from build123d import *

# Parameters (mm, degrees)
BOSS_EXTRUDE1_DEPTH     = 40
CUT_EXTRUDE1_DEPTH      = 13
CUT_EXTRUDE1_DEPTH_BACK = 50
SKETCH12_R              = 1.150000001
SKETCH14_R              = 1.150000001
CUT_EXTRUDE2_DEPTH      = 50
SKETCH15_R              = 1.150000001
CUT_EXTRUDE3_DEPTH      = 50
SKETCH18_R              = 7.063467882
CUT_EXTRUDE6_DEPTH      = 50
CUT_EXTRUDE8_DEPTH      = 50
CUT_EXTRUDE8_DEPTH_BACK = 50
SKETCH19_R              = 1.6
SKETCH19_R_2            = 2.999999999


with BuildPart() as part:
    # Sketch9 → Boss-Extrude1 (new body)
    with BuildSketch(Plane(origin=(23635.895639599, 0, 0), x_dir=(0, 0, -1), z_dir=(1, 0, 0))):
        with BuildLine():
            Line((44.099999999, 2015.086397777), (44.099999999, 2022.286397779))
            Line((44.099999999, 2022.286397779), (42.3, 2022.286397779))
            Line((42.3, 2022.286397779), (42.3, 2015.286397778))
            ThreePointArc((42.3, 2015.286397778), (42.007106781, 2014.579290998), (41.300000001, 2014.286397779))
            Line((41.300000001, 2014.286397779), (2.800000001, 2014.286397779))
            ThreePointArc((2.800000001, 2014.286397779), (2.092893219, 2014.579290997), (1.799999999, 2015.286397778))
            Line((1.799999999, 2015.286397778), (1.799999999, 2022.286397779))
            Line((1.799999999, 2022.286397779), (0, 2022.286397779))
            Line((0, 2022.286397779), (0, 2015.086397777))
            ThreePointArc((0, 2015.086397777), (0.761522369, 2013.247920146), (2.599999999, 2012.486397778))
            Line((2.599999999, 2012.486397778), (41.5, 2012.486397778))
            ThreePointArc((41.5, 2012.486397778), (43.33847763, 2013.247920146), (44.099999999, 2015.086397777))
        make_face()
    extrude(amount=-BOSS_EXTRUDE1_DEPTH)

    # Sketch12 → Cut-Extrude1 (cut, two sides: drawn at the far end of the back side and taken through both)
    with BuildSketch(Plane.XY.offset(-CUT_EXTRUDE1_DEPTH_BACK)):
        with Locations(Location((23613.365202112, 2019.805962196, 0), (0, 0, 180))):
            Circle(SKETCH12_R)
    extrude(amount=CUT_EXTRUDE1_DEPTH + CUT_EXTRUDE1_DEPTH_BACK, mode=Mode.SUBTRACT)

    # Sketch14 → Cut-Extrude2 (cut)
    with BuildSketch(Plane.XY):
        with Locations((23605.845202113, 2020.305962197)):
            Circle(SKETCH14_R)
    extrude(amount=-CUT_EXTRUDE2_DEPTH, mode=Mode.SUBTRACT)

    # Sketch15 → Cut-Extrude3 (cut)
    with BuildSketch(Plane.XY):
        with Locations((23598.365202112, 2019.805962196)):
            Circle(SKETCH15_R)
    extrude(amount=-CUT_EXTRUDE3_DEPTH, mode=Mode.SUBTRACT)

    # Sketch18 → Cut-Extrude6 (cut)
    with BuildSketch(Plane.XY):
        with Locations((23625.865202113, 2027.305962196)):
            Circle(SKETCH18_R)
    extrude(amount=-CUT_EXTRUDE6_DEPTH, mode=Mode.SUBTRACT)

    # Sketch19 → Cut-Extrude8 (cut, two sides: drawn at the far end of the back side and taken through both)
    with BuildSketch(Plane(origin=(0, 2012.486397778, 0), x_dir=(-1, 0, 0), z_dir=(0, 1, 0)).offset(-CUT_EXTRUDE8_DEPTH_BACK)):
        with Locations(Location((-23605.996144663, -8.550000002, 0), (0, 0, 269.999999999))):
            Circle(SKETCH19_R)
        with Locations(Location((-23615.895639599, -8.550000002, 0), (0, 0, 269.999999999))):
            Circle(SKETCH19_R)
        with Locations(Location((-23625.795134534, -8.550000002, 0), (0, 0, 269.999999999))):
            Circle(SKETCH19_R)
        with Locations(Location((-23630.744882003, -17.100252533, 0), (0, 0, 270))):
            Circle(SKETCH19_R)
        with Locations(Location((-23620.845387068, -17.100252533, 0), (0, 0, 269.999999999))):
            Circle(SKETCH19_R)
        with Locations(Location((-23610.94589213, -17.100252533, 0), (0, 0, 269.999999999))):
            Circle(SKETCH19_R)
        with Locations(Location((-23601.046397194, -17.100252533, 0), (0, 0, 269.999999999))):
            Circle(SKETCH19_R)
        with Locations(Location((-23601.046397194, -26.999747469, 0), (0, 0, 269.999999999))):
            Circle(SKETCH19_R)
        with Locations(Location((-23610.94589213, -26.999747469, 0), (0, 0, 269.999999999))):
            Circle(SKETCH19_R)
        with Locations(Location((-23620.845387068, -26.999747469, 0), (0, 0, 269.999999999))):
            Circle(SKETCH19_R)
        with Locations(Location((-23630.744882003, -26.999747469, 0), (0, 0, 270))):
            Circle(SKETCH19_R)
        with Locations(Location((-23625.795134534, -35.550000002, 0), (0, 0, 269.999999999))):
            Circle(SKETCH19_R)
        with Locations(Location((-23615.895639599, -35.550000002, 0), (0, 0, 269.999999999))):
            Circle(SKETCH19_R)
        with Locations(Location((-23605.996144663, -35.550000002, 0), (0, 0, 269.999999999))):
            Circle(SKETCH19_R)
        with Locations(Location((-23615.895639599, -22.050000002, 0), (0, 0, 270))):
            Circle(SKETCH19_R_2)
        with Locations(Location((-23625.795134534, -22.050000002, 0), (0, 0, 270))):
            Circle(SKETCH19_R_2)
        with Locations(Location((-23605.996144663, -22.050000002, 0), (0, 0, 269.999999999))):
            Circle(SKETCH19_R_2)
    extrude(amount=CUT_EXTRUDE8_DEPTH + CUT_EXTRUDE8_DEPTH_BACK, mode=Mode.SUBTRACT)


solid = part.part
Model file for the job. Use its own axes, mm. A direction names the side the tool comes from. Give positions to 0.01 mm unless a question says otherwise; leave off trailing zeros. Order: outer loops, then holes, each group sorted by start corner. A loop starts at its lowest first (then second) coordinate and runs counter-clockwise, first axis right, second up. Notation, with made-up numbers: M -8,29 L 10,29 A38 ccw 10,68 Z; hole C 57,-19.5 d3. An arc over 180 degrees is marked long. Write item = value, one per line.
Q1. Cut at B-B, the plane y = 2016.5. List the corners of the cut face in (x, z).
Derived:
outline = M 23595.9,-44.1 L 23635.9,-44.1 L 23635.9,-42.3 L 23595.9,-42.3 Z; M 23595.9,-1.8 L 23635.9,-1.8 L 23635.9,0 L 23595.9,0 Z
Q2. Cut at C-C, the plane x = 23600.5. List the corners of the cut face in (y, z), then the cut area to 3 significant figures.
Derived:
outline = M 2012.49,-41.5 A2.6 ccw 2015.09,-44.1 L 2022.29,-44.1 L 2022.29,-42.3 L 2015.29,-42.3 A1 cw 2014.29,-41.3 L 2014.29,-28.5 L 2012.49,-28.5 Z; M 2012.49,-25.5 L 2014.29,-25.5 L 2014.29,-18.6 L 2012.49,-18.6 Z; M 2012.49,-15.6 L 2014.29,-15.6 L 2014.29,-2.8 A1 cw 2015.29,-1.8 L 2022.29,-1.8 L 2022.29,0 L 2015.09,0 A2.6 ccw 2012.49,-2.6 Z
area = 94.9 mm2
Q3. Cut at A-A, the plane z = -35.55. List the corners of the cut face in (x, y).
Derived:
outline = M 23595.9,2012.49 L 23604.4,2012.49 L 23604.4,2014.29 L 23595.9,2014.29 Z; M 23607.6,2012.49 L 23614.3,2012.49 L 23614.3,2014.29 L 23607.6,2014.29 Z; M 23617.5,2012.49 L 23624.2,2012.49 L 23624.2,2014.29 L 23617.5,2014.29 Z; M 23627.4,2012.49 L 23635.9,2012.49 L 23635.9,2014.29 L 23627.4,2014.29 Z
Q4. Drill centre lines: line 1 (X direction, y = 2013.4, z = -8.55); line 2 (X direction, y = 2013, z = -22.05); line 3 (Z direction, x = 23610, y = 2018.75). Where is each one in solid material? Low to high. Write a range as [from, to].
Derived:
line_1 = [23595.9, 23604.4], [23607.6, 23614.3], [23617.5, 23624.2], [23627.4, 23635.9]
line_2 = [23595.9, 23603], [23609, 23612.9], [23618.9, 23622.8], [23628.8, 23635.9]
line_3 = [-44.1, -42.3], [-1.8, 0]
Q5. Cut at D-D, the plane x = 23618. List the corners of the cut face in (y, z), then the cut area to 3 significant figures.
Derived:
outline = M 2012.49,-41.5 A2.6 ccw 2015.09,-44.1 L 2022.29,-44.1 L 2022.29,-42.3 L 2015.29,-42.3 A1 cw 2014.29,-41.3 L 2014.29,-24.19 L 2012.49,-24.19 Z; M 2012.49,-19.91 L 2014.29,-19.91 L 2014.29,-2.8 A1 cw 2015.29,-1.8 L 2022.29,-1.8 L 2022.29,0 L 2015.09,0 A2.6 ccw 2012.49,-2.6 Z
area = 98.0 mm2
Q6. Tool access for faces 1 (the cylindrical face through (23617.458, 2013.374, -35.203)), 2 (the flat face through (23616, 2019, -42.3)): list every direction of +Z, -Z, +X, -X, +Y, -Y with a clear straight run to the whole face (end or side of a thin tool).
Derived:
face_1 = +Y, -Y
face_2 = +X, -X, +Y
Q7. Flat gauge pin, fed straight in: pin 1 (4 mm diameter, centred on x = 23606, z = -8.55, fed in from +Y). Where does the tip first touch, or does it go through?
Derived:
pin_1 = 2014.29
Q8. Two-plate mould, pull along Z, no slides. Class faces 3 (the cylindrical face through (23599.462, 2020.151, -0.887)), 4 (the flat face through (23616, 2019, -1.8)), 5 (the cylindrical face through (23603.02, 2013.37, -21.66)): pulls with the +Z half, pulls with the -Z half, needs draft (parallel to the pull), parting line crosses it, or undercut.
Derived:
face_3 = needs draft
face_4 = undercut
face_5 = undercut
